The listing builds one solid part. Answer for the finished solid, in the listing's coordinates (mm). Round coordinates to 2 decimals unless told otherwise and drop trailing zeros. Order: outer loops, then holes, each group sorted by start corner. A loop starts at its lowest first (then second) coordinate and runs counter-clockwise, first axis right, second up. Notation, with made-up numbers: (60, 28) -> (67, 28) arc R32 ccw to (67, 56) -> close; hole circle Ø8 at (85, 10.5). An arc over 180 degrees is marked (long way). Return JSON: item names as keys, results as strings. Group by question number.
(1) Each of these flat-tipped pins is pushed along its axis until it touches: pin 1 (2 mm diameter, centred on x = 13, y = -0.5, fed in from +Z); pin 2 (6 mm diameter, centred on x = -6.5, y = 4, fed in from +Z); pin 3 (6 mm diameter, centred on x = 2, y = 0, fed in from -Z). Where does it stop, or does it pass through?
(2) The part is cut by section B-B (x = -4). Determine the outline of the cut face in (y, z), plus the area to 3 significant figures.
(3) The part is cut by section A-A (y = -4.25). Determine the outline of the cut face in (x, z).
(4) Consider line 1 (Y direction, x = -0.5, z = 27); line 2 (X direction, y = 1.75, z = 13); line 3 (X direction, y = -1, z = -18). Determine where each line is inside the solid, lowest interval first. Write a range as [from, to].
(5) The part is cut by section C-C (z = -2). Determine the outline of the cut face in (x, y).
(6) The part is cut by section D-D (z = 23.5). Determine the outline of the cut face in (x, y), plus the area to 3 significant figures.
(7) Determine the mould class of faces 1 (the face through (29.97, 3.98, -1.32)), 2 (the face through (-7, -5.5, -18)), 3 (the face through (9.18, 0.08, -17.43)) for opening direction Z: +Z half, -Z half, draft (parallel to the pull), parting line (faces both ways), or undercut.
from build123d import *

# Parameters (mm, degrees)
CUT_EXTRUDE1_REACH = 13


with BuildPart() as part:
    # Sketch2 → Revolve1 (revolve)
    with BuildSketch(Plane.XY):
        Polygon((-25, 2.5), (-25, -2.5), (-30, -2.5), (-30, -5.5), (0, -5.5), (0, 5.5), (-30, 5.5), (-30, 2.5), align=None)
    revolve(axis=Axis((0, 19.987411147, 0), (0, -1, 0)))

    # Sketch3 → Cut-Extrude1 (cut, up to next)
    with BuildSketch(Plane(origin=(0, 5.5, 0), x_dir=(1, 0, 0), z_dir=(0, 1, 0)), mode=Mode.PRIVATE) as cut_extrude1_sk1:
        with BuildLine():
            ThreePointArc((15.256177825, -16.943702021), (19.745379206, -11.4), (22.301765297, -4.740386551))
            Line((22.301765297, -4.740386551), (16.139435412, -3.430542898))
            ThreePointArc((16.139435412, -3.430542898), (16.372933017, -2.043786781), (16.487498259, -0.642184674))
            Line((16.487498259, -0.642184674), (22.782724867, -0.887382459))
            ThreePointArc((22.782724867, -0.887382459), (19.745379206, 11.4), (10.622866681, 20.174109732))
            Line((10.622866681, 20.174109732), (7.687600888, 14.599684674))
            ThreePointArc((7.687600888, 14.599684674), (6.416495236, 15.201269318), (5.098780407, 15.692432519))
            Line((5.098780407, 15.692432519), (7.045587472, 21.684088572))
            ThreePointArc((7.045587472, 21.684088572), (0, 22.8), (-7.045587472, 21.684088572))
            Line((-7.045587472, 21.684088572), (-5.098780407, 15.692432519))
            ThreePointArc((-5.098780407, 15.692432519), (-6.416495236, 15.201269318), (-7.687600888, 14.599684674))
            Line((-7.687600888, 14.599684674), (-10.622866681, 20.174109732))
            ThreePointArc((-10.622866681, 20.174109732), (-19.745379206, 11.4), (-22.782724867, -0.887382459))
            Line((-22.782724867, -0.887382459), (-16.487498259, -0.642184674))
            ThreePointArc((-16.487498259, -0.642184674), (-16.372933017, -2.043786781), (-16.139435412, -3.430542898))
            Line((-16.139435412, -3.430542898), (-22.301765297, -4.740386551))
            ThreePointArc((-22.301765297, -4.740386551), (-19.745379206, -11.4), (-15.256177825, -16.943702021))
            Line((-15.256177825, -16.943702021), (-11.040655005, -12.26188962))
            ThreePointArc((-11.040655005, -12.26188962), (-9.956437781, -13.157482537), (-8.799897372, -13.9575))
            Line((-8.799897372, -13.9575), (-12.159858186, -19.286727273))
            ThreePointArc((-12.159858186, -19.286727273), (0, -22.8), (12.159858186, -19.286727273))
            Line((12.159858186, -19.286727273), (8.799897372, -13.9575))
            ThreePointArc((8.799897372, -13.9575), (9.956437781, -13.157482537), (11.040655005, -12.26188962))
            Line((11.040655005, -12.26188962), (15.256177825, -16.943702021))
        make_face()
    cut_extrude1_tool1 = extrude(cut_extrude1_sk1.sketch, amount=-CUT_EXTRUDE1_REACH, mode=Mode.PRIVATE) & part.part
    add(cut_extrude1_tool1.solids().sort_by_distance((0, 5.5, 0))[0], mode=Mode.SUBTRACT)


solid = part.part
Answer below:
{
 "1": {"pin 1": "stops at z = 21.93", "pin 2": "stops at z = 29.8", "pin 3": "stops at z = -30"},
 "2": {"outline": "(-5.5, -29.73) -> (-2.5, -29.73) -> (-2.5, -24.68) -> (2.5, -24.68) -> (2.5, -29.73) -> (5.5, -29.73) -> (5.5, -22.45) -> (-5.5, -22.45) -> close; (-5.5, 22.45) -> (5.5, 22.45) -> (5.5, 29.73) -> (2.5, 29.73) -> (2.5, 24.68) -> (-2.5, 24.68) -> (-2.5, 29.73) -> (-5.5, 29.73) -> close", "area": "110 mm²"},
 "3": {"outline": "circle Ø60 at (0, 0); hole (-22.78, 0.89) arc R22.8 ccw to (-10.62, -20.17) -> (-7.69, -14.6) arc R16.5 ccw to (-5.1, -15.69) -> (-7.05, -21.68) arc R22.8 ccw to (7.05, -21.68) -> (5.1, -15.69) arc R16.5 ccw to (7.69, -14.6) -> (10.62, -20.17) arc R22.8 ccw to (22.78, 0.89) -> (16.49, 0.64) arc R16.5 ccw to (16.14, 3.43) -> (22.3, 4.74) arc R22.8 ccw to (15.26, 16.94) -> (11.04, 12.26) arc R16.5 ccw to (8.8, 13.96) -> (12.16, 19.29) arc R22.8 ccw to (-12.16, 19.29) -> (-8.8, 13.96) arc R16.5 ccw to (-11.04, 12.26) -> (-15.26, 16.94) arc R22.8 ccw to (-22.3, 4.74) -> (-16.14, 3.43) arc R16.5 ccw to (-16.49, 0.64) -> close"},
 "4": {"line 1": "y = [-5.5, -2.5], [2.5, 5.5]", "line 2": "x = [-21.35, -18.73], [-11.71, -10.16], [10.16, 11.71], [18.73, 21.35]", "line 3": "x = [-17.35, -13.99], [-9.48, -5.85], [5.85, 9.48], [13.99, 17.35]"},
 "5": {"outline": "(-29.93, -5.5) -> (-22.71, -5.5) -> (-22.71, 5.5) -> (-29.93, 5.5) -> (-29.93, 2.5) -> (-24.92, 2.5) -> (-24.92, -2.5) -> (-29.93, -2.5) -> close; (22.71, -5.5) -> (29.93, -5.5) -> (29.93, -2.5) -> (24.92, -2.5) -> (24.92, 2.5) -> (29.93, 2.5) -> (29.93, 5.5) -> (22.71, 5.5) -> close"},
 "6": {"outline": "(-18.65, -5.5) -> (18.65, -5.5) -> (18.65, -2.5) -> (8.53, -2.5) -> (8.53, 2.5) -> (18.65, 2.5) -> (18.65, 5.5) -> (-18.65, 5.5) -> (-18.65, 2.5) -> (-8.53, 2.5) -> (-8.53, -2.5) -> (-18.65, -2.5) -> close", "area": "309 mm²"},
 "7": {"face 1": "parting line", "face 2": "draft", "face 3": "undercut"}
}
